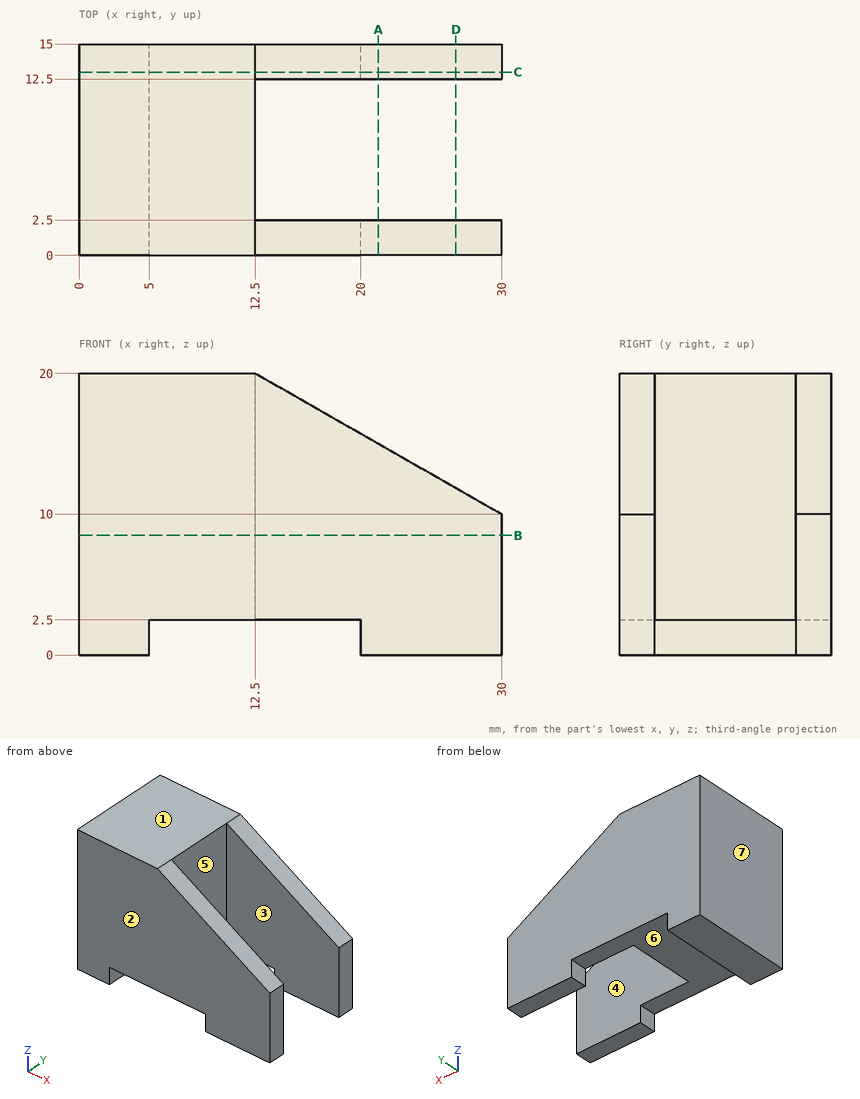
Geometry: see drawing. Coordinates: mm, zero at the bounding-box minimum. A direction names the side the tool comes from. Round coordinates to 2 decimals unless told otherwise and drop trailing zeros. Write each loop counter-clockwise with the first axis right and the second up, starting at its lowest first coordinate (ties: lowest second). Pieces come first, ordered by that corner, then holes. Notation, with made-up numbers: M -0.75,-21 L 32.25,-21 A9 cw 32.25,-12 Z; hole C 80.5,33.25 d3. An arc over 180 degrees is marked long. Answer in a Markdown table with one row per item. Add a question column.
(1) Ray query, L1, parallel to Y at x = 16.75, z = 5; L2, parallel to X at y = 8, z = 7.5; L3, parallel to Z at x = 10.5, y = 10. Return the intervals inside material, ascending.
(2) Cut plane D-D, the plane x = 26.75. Return the cut outline in (y, z).
(3) Cut plane B-B, the plane z = 8.5. Return the cut outline in (x, y), then the cut area to 3 significant figures.
(4) Contact query for flat-ended pins moving along their axis: pin 1 (1 mm diameter, centred on x = 16.5, z = 10.5, fed in from -Y); pin 2 (5 mm diameter, centred on y = 6.5, z = 12.5, fed in from +X); pin 3 (0.8 mm diameter, centred on y = 5, z = 1, fed in from +X). Output: stop coordinate, or through.
(5) Cut plane C-C, the plane y = 13. Return the cut outline in (x, z), then the cut area to 3 significant figures.
(6) Cut plane A-A, the plane x = 21.25. Return the cut outline in (y, z).
(7) Draft query along Y for the marked faces 1, 2, 3 and 4. Return one class per face: pulls with the +Y half, pulls with the -Y half, needs draft (parallel to the pull), parting line crosses it, or undercut.
(8) Reachability of the marked faces 5, 6 and 7 from +Z, -Z, +X, -X, +Y, -Y: full face, straight path, thin tool, end or side. Return the list, or none.
Established:
| question | item | result |
|---|---|---|
| 1 | L1 | 0 to 2.5, 12.5 to 15 |
| 1 | L2 | 0 to 12.5 |
| 1 | L3 | 2.5 to 20 |
| 2 | outline | M 0,0 L 2.5,0 L 2.5,11.86 L 0,11.86 Z; M 12.5,0 L 15,0 L 15,11.86 L 12.5,11.86 Z |
| 3 | outline | M 0,0 L 30,0 L 30,2.5 L 12.5,2.5 L 12.5,12.5 L 30,12.5 L 30,15 L 0,15 Z |
| 3 | area | 275 mm² |
| 4 | pin 1 | y = 0 |
| 4 | pin 2 | x = 12.5 |
| 4 | pin 3 | x = 5 |
| 5 | outline | M 0,0 L 5,0 L 5,2.5 L 20,2.5 L 20,0 L 30,0 L 30,10 L 12.5,20 L 0,20 Z |
| 5 | area | 475 mm² |
| 6 | outline | M 0,0 L 2.5,0 L 2.5,15 L 0,15 Z; M 12.5,0 L 15,0 L 15,15 L 12.5,15 Z |
| 7 | face 1 | needs draft |
| 7 | face 2 | pulls with the -Y half |
| 7 | face 3 | undercut |
| 7 | face 4 | undercut |
| 8 | face 5 | +Z, -Z, +X |
| 8 | face 6 | -Z, +Y, -Y |
| 8 | face 7 | +Z, -Z, -X, +Y, -Y |
